```python
from build123d import *

# Parameters (mm, degrees)
SZKIC6_R                    = 12.7
DODANIE_WYCI_GNI_CIE3_DEPTH = 3
SZKIC7_W                    = 8
SZKIC7_H                    = 2
ZAOKR_GLENIE3_R             = 4


with BuildPart() as part:
    # Szkic5 → Obrót1 (revolve)
    with BuildSketch(Plane.XY):
        with BuildLine():
            Line((0, 6.35), (1, 6.35))
            ThreePointArc((1, 6.35), (2, 5.35), (3, 6.35))
            Line((3, 6.35), (3, 0))
            Line((3, 0), (0, 0))
            Line((0, 0), (-9, 0))
            Line((-9, 0), (-9, 4.35))
            Line((-9, 4.35), (0, 4.35))
            Line((0, 4.35), (0, 6.35))
        make_face()
    revolve(axis=Axis((0, 0, 0), (-1, 0, 0)))

    # Szkic6 → Dodanie-wyciągnięcie3 (add)
    with BuildSketch(Plane(origin=(3, 0, 0), x_dir=(0, 0, -1), z_dir=(1, 0, 0))):
        with Locations(Location((0, 0, 0), (0, 0, 90))):
            Circle(SZKIC6_R)
    extrude(amount=DODANIE_WYCI_GNI_CIE3_DEPTH)

    # Wyciągnięcie po ścieżce1: sweep along a path in Szkic1
    with BuildLine(Plane.XY) as wyci_gni_cie_po_cie_ce1_path:
        Line((110, 5), (110, 15))
        ThreePointArc((110, 15), (135.606601718, 25.606601718), (125, 0))
        Line((125, 0), (0, 0))
        Line((0, 0), (-520, 0))
        Line((-520, 0), (-523, 3))
        Line((-523, 3), (-537, 3))
        Line((-537, 3), (-540, 0))
        Line((-540, 0), (-555, 0))
    # Szkic7 → Wyciągnięcie po ścieżce1 (sweep)
    with BuildSketch(Plane(origin=(0, 0, 0), x_dir=(0, 0, -1), z_dir=(1, 0, 0))):
        Rectangle(SZKIC7_W, SZKIC7_H)
    sweep(path=wyci_gni_cie_po_cie_ce1_path.line, transition=Transition.RIGHT)

    # Zaokrąglenie3
    zaokr_glenie3_edges = [part.edges().sort_by_distance(p)[0] for p in [
        (-555, 0, -4),
        (-555, 0, 4),
    ]]
    fillet(zaokr_glenie3_edges, radius=ZAOKR_GLENIE3_R - 0.0001)  # a hair under: the kernel refuses the full size


solid = part.part
```
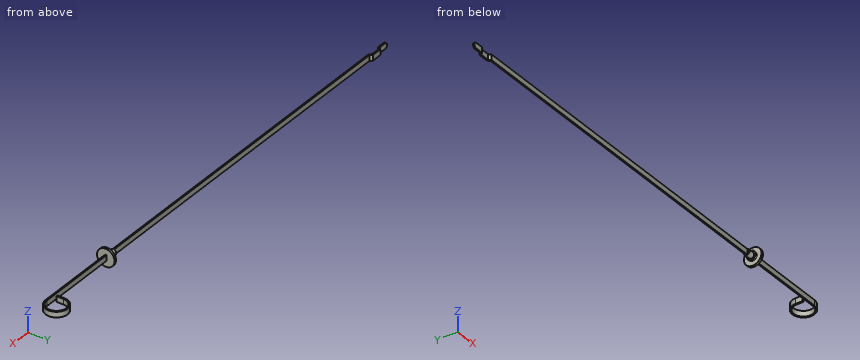
Geometry: final body of the model. Coordinates: model frame, mm. Coordinates: 2 decimals unless noted, no trailing zeros. Order: outer loops, then holes, each group sorted by start corner. A loop starts at its lowest first (then second) coordinate and runs counter-clockwise, first axis right, second up. Notation, with made-up numbers: (57.5, 62.5) -> (78.5, 62.5) arc R27 ccw to (78.5, 99.5) -> close; hole circle Ø3 at (79, -35). An arc over 180 degrees is marked (long way). Use CSV: the item, a comma, the result in double quotes.
1) Section A-A on x = -112. Output: boundary loops of the cut face in (y, z).
Findings:
outline,"(-1, -4) -> (1, -4) -> (1, 4) -> (-1, 4) -> close"
2) Line query: line 1 (Y direction, x = 125, z = 1.75); line 2 (Y direction, x = -14.5, z = 1.5); line 3 (X direction, y = 18.5, z = -1). Output: solid intervals per line, ascending.
Findings:
line 1,"y = -1 to 1, 29 to 31"
line 2,"y = -1 to 1"
line 3,"x = 109.39 to 111.44, 138.56 to 140.61"
3) Pin query (flat end, axial travel): pin 1 Ø6 at (x, z) = (-404, 0) entering from +Y; pin 2 Ø9 at (x, z) = (-527, 1.5) entering from -Y; pin 3 Ø5.5 at (x, y) = (-189, 2.5) entering from -Z. Return the tip coordinate at first contact, or that it passes through.
Findings:
pin 1,"stops at y = 1"
pin 2,"stops at y = 1.09"
pin 3,"stops at z = -4"
